from build123d import *

# Parameters (mm, degrees)
BRIDA_BASE1_DEPTH                   = 2.5
CROQUIS16_W                         = 1.5
CROQUIS16_H                         = 11
CORTAR_EXTRUIR1_DEPTH               = 48.758002549
CROQUIS17_W                         = 1.5
CROQUIS17_H                         = 11
CORTAR_EXTRUIR2_DEPTH               = 48.758002549
CROQUIS18_R                         = 2
SALIENTE_EXTRUIR1_DEPTH             = 1.5
CROQUIS19_R                         = 2.7
SALIENTE_EXTRUIR2_DEPTH             = 4.5
CROQUIS20_R                         = 2.7
SALIENTE_EXTRUIR3_DEPTH             = 4.5
CROQUIS21_R                         = 2
SALIENTE_EXTRUIR4_DEPTH             = 1.5
DI_METRO_DE_TALADRO_3_0_3_1_D       = 3
DI_METRO_DE_TALADRO_3_0_3_2_D       = 3
DI_METRO_DE_TALADRO_3_0_3_2_DEPTH   = 8.5
DI_METRO_DE_TALADRO_7_2_7_2_1_D     = 7.2
DI_METRO_DE_TALADRO_7_2_7_2_1_DEPTH = 4
DI_METRO_DE_TALADRO_3_0_3_3_D       = 3
DI_METRO_DE_TALADRO_3_0_3_3_DEPTH   = 8.5
DI_METRO_DE_TALADRO_5_0_5_1_D       = 5
DI_METRO_DE_TALADRO_5_0_5_1_DEPTH   = 7
PLIEGUE_START                       = -35.363495408
PLIEGUE_CROQUIZADO1_OUTLINE_W       = 17
PLIEGUE_CROQUIZADO1_OUTLINE_H       = 2.5
PLIEGUE_CROQUIZADO1_DEPTH           = 19.863495408
PLIEGUE_START_2                     = -15.5
PLIEGUE_CROQUIZADO1_2_DEPTH         = 2.5
PLIEGUE_START_3                     = 15
PLIEGUE_CROQUIZADO1_3_DEPTH         = 18
PLIEGUE_CROQUIZADO2_OUTLINE_W       = 17
PLIEGUE_CROQUIZADO2_OUTLINE_H       = 2.5
PLIEGUE_CROQUIZADO2_DEPTH           = 19.863495408
PLIEGUE_CROQUIZADO2_2_DEPTH         = 2.5
PLIEGUE_START_4                     = -33
PLIEGUE_CROQUIZADO2_3_DEPTH         = 18


with BuildPart() as part:
    # Brida base1: sheet metal written as solids
    # Croquis11 → Brida base1 (new body)
    with BuildSketch(Plane.XY.offset(2.5)):
        with BuildLine():
            Line((-30, -35.363495408), (-17, -35.363495408))
            ThreePointArc((-17, -35.363495408), (-15.585786438, -34.777708971), (-15, -33.363495408))
            Line((-15, -33.363495408), (-15, -12.875))
            Line((-15, -12.875), (-14.875, -12.875))
            Line((-14.875, -12.875), (-14.875, -15.5))
            Line((-14.875, -15.5), (-12, -15.5))
            Line((-12, -15.5), (-12, -20))
            ThreePointArc((-12, -20), (0, -32), (12, -20))
            Line((12, -20), (12, -15.5))
            Line((12, -15.5), (14.875, -15.5))
            Line((14.875, -15.5), (14.875, -12.875))
            Line((14.875, -12.875), (15, -12.875))
            Line((15, -12.875), (15, -33.363495408))
            ThreePointArc((15, -33.363495408), (15.585786438, -34.777708971), (17, -35.363495408))
            Line((17, -35.363495408), (30, -35.363495408))
            ThreePointArc((30, -35.363495408), (31.414213562, -34.777708971), (32, -33.363495408))
            Line((32, -33.363495408), (32, 22))
            ThreePointArc((32, 22), (29.071067812, 29.071067812), (22, 32))
            Line((22, 32), (-22, 32))
            ThreePointArc((-22, 32), (-29.071067812, 29.071067812), (-32, 22))
            Line((-32, 22), (-32, -33.363495408))
            ThreePointArc((-32, -33.363495408), (-31.414213562, -34.777708971), (-30, -35.363495408))
        make_face()
    extrude(amount=-BRIDA_BASE1_DEPTH)

    # Croquis16 → Cortar-Extruir1 (cut, through all)
    with BuildSketch(Plane.XY.offset(2.5)):
        with Locations((-20.75, -29.863495408)):
            Rectangle(CROQUIS16_W, CROQUIS16_H)
    extrude(amount=-CORTAR_EXTRUIR1_DEPTH, mode=Mode.SUBTRACT)

    # Croquis17 → Cortar-Extruir2 (cut, through all)
    with BuildSketch(Plane(origin=(0, 0, 0), x_dir=(-1, 0, 0), z_dir=(0, 0, -1))):
        with Locations((-20.75, -29.863495408)):
            Rectangle(CROQUIS17_W, CROQUIS17_H)
    extrude(amount=-CORTAR_EXTRUIR2_DEPTH, mode=Mode.SUBTRACT)

    # Croquis18 → Saliente-Extruir1 (add)
    with BuildSketch(Plane(origin=(0, 0, 0), x_dir=(-1, 0, 0), z_dir=(0, 0, -1))):
        with Locations(Location((1.5, 17.65, 0), (0, 0, 180))):
            Circle(CROQUIS18_R)
    extrude(amount=SALIENTE_EXTRUIR1_DEPTH)

    # Croquis19 → Saliente-Extruir2 (add)
    with BuildSketch(Plane.XY.offset(2.5)):
        with Locations((23.5, 7.55)):
            Circle(CROQUIS19_R)
    extrude(amount=SALIENTE_EXTRUIR2_DEPTH)

    # Croquis20 → Saliente-Extruir3 (add)
    with BuildSketch(Plane.XY.offset(2.5)):
        with Locations((9.5, 7.55)):
            Circle(CROQUIS20_R)
    extrude(amount=SALIENTE_EXTRUIR3_DEPTH)

    # Croquis21 → Saliente-Extruir4 (add)
    with BuildSketch(Plane(origin=(0, 0, 0), x_dir=(-1, 0, 0), z_dir=(0, 0, -1))):
        with Locations(Location((19, -1.25, 0), (0, 0, 180))):
            Circle(CROQUIS21_R)
    extrude(amount=SALIENTE_EXTRUIR4_DEPTH)

    # Diámetro de taladro Ø3.0 (3)1 (through all)
    with Locations(Plane.XY.offset(2.5)):
        with Locations((-19, -1.25)):
            Hole(DI_METRO_DE_TALADRO_3_0_3_1_D / 2)

    # Diámetro de taladro Ø3.0 (3)2
    with Locations(Plane.XY.offset(7)):
        with Locations((23.5, 7.55), (9.5, 7.55)):
            Hole(DI_METRO_DE_TALADRO_3_0_3_2_D / 2, depth=DI_METRO_DE_TALADRO_3_0_3_2_DEPTH)

    # Diámetro de taladro Ø7.2 (7.2)1
    with Locations(Plane.XY.offset(2.5)):
        with Locations((0, -20.1)):
            Hole(DI_METRO_DE_TALADRO_7_2_7_2_1_D / 2, depth=DI_METRO_DE_TALADRO_7_2_7_2_1_DEPTH)

    # Diámetro de taladro Ø3.0 (3)3
    with Locations(Plane(origin=(0, 0, -1.5), x_dir=(-1, 0, 0), z_dir=(0, 0, -1))):
        with Locations((1.5, 17.65)):
            Hole(DI_METRO_DE_TALADRO_3_0_3_3_D / 2, depth=DI_METRO_DE_TALADRO_3_0_3_3_DEPTH)

    # Diámetro de taladro Ø5.0 (5)1
    with Locations(Plane(origin=(0, 0, 0), x_dir=(-1, 0, 0), z_dir=(0, 0, -1))):
        with Locations((20, 20.1), (-20, 20.1)):
            Hole(DI_METRO_DE_TALADRO_5_0_5_1_D / 2, depth=DI_METRO_DE_TALADRO_5_0_5_1_DEPTH)

    # Pliegue croquizado1: read off the stored shape, not the designer's step
    # Pliegue croquizado1 outline → Pliegue croquizado1 (cut)
    with BuildSketch(Plane(origin=(0, 0, 0), x_dir=(1, 0, 0), z_dir=(0, 1, 0)).offset(PLIEGUE_START)):
        with Locations((23.5, -1.25)):
            Rectangle(PLIEGUE_CROQUIZADO1_OUTLINE_W, PLIEGUE_CROQUIZADO1_OUTLINE_H)
    extrude(amount=PLIEGUE_CROQUIZADO1_DEPTH, mode=Mode.SUBTRACT)

    # Pliegue croquizado1 2 outline → Pliegue croquizado1 2 (add)
    with BuildSketch(Plane(origin=(0, 0, 0), x_dir=(1, 0, 0), z_dir=(0, 1, 0)).offset(PLIEGUE_START_2)):
        with BuildLine():
            Line((15, 0), (32, 0))
            Line((32, 0), (32, 18.4))
            ThreePointArc((32, 18.4), (31.414213562, 19.814213562), (30, 20.4))
            Line((30, 20.4), (21.5, 20.4))
            Line((21.5, 20.4), (21.5, 9.4))
            Line((21.5, 9.4), (20, 9.4))
            Line((20, 9.4), (20, 20.4))
            Line((20, 20.4), (17, 20.4))
            ThreePointArc((17, 20.4), (15.585786438, 19.814213562), (15, 18.4))
            Line((15, 18.4), (15, 0))
        make_face()
    extrude(amount=PLIEGUE_CROQUIZADO1_2_DEPTH)

    # Pliegue croquizado1 3 outline → Pliegue croquizado1 3 (cut)
    with BuildSketch(Plane.YZ.offset(PLIEGUE_START_3)):
        with BuildLine():
            Line((-15.5, 2.5), (-15.5, 0))
            ThreePointArc((-15.5, 0), (-14.767766953, 1.767766953), (-13, 2.5))
            Line((-13, 2.5), (-15.5, 2.5))
        make_face()
    extrude(amount=PLIEGUE_CROQUIZADO1_3_DEPTH, mode=Mode.SUBTRACT)

    # Pliegue croquizado2: read off the stored shape, not the designer's step
    # Pliegue croquizado2 outline → Pliegue croquizado2 (cut)
    with BuildSketch(Plane(origin=(0, 0, 0), x_dir=(1, 0, 0), z_dir=(0, 1, 0)).offset(PLIEGUE_START)):
        with Locations((-23.5, -1.25)):
            Rectangle(PLIEGUE_CROQUIZADO2_OUTLINE_W, PLIEGUE_CROQUIZADO2_OUTLINE_H)
    extrude(amount=PLIEGUE_CROQUIZADO2_DEPTH, mode=Mode.SUBTRACT)

    # Pliegue croquizado2 2 outline → Pliegue croquizado2 2 (add)
    with BuildSketch(Plane(origin=(0, 0, 0), x_dir=(1, 0, 0), z_dir=(0, 1, 0)).offset(PLIEGUE_START_2)):
        with BuildLine():
            ThreePointArc((-30, 20.4), (-31.414213562, 19.814213562), (-32, 18.4))
            Line((-32, 18.4), (-32, 0))
            Line((-32, 0), (-15, 0))
            Line((-15, 0), (-15, 18.4))
            ThreePointArc((-15, 18.4), (-15.585786438, 19.814213562), (-17, 20.4))
            Line((-17, 20.4), (-20, 20.4))
            Line((-20, 20.4), (-20, 9.4))
            Line((-20, 9.4), (-21.5, 9.4))
            Line((-21.5, 9.4), (-21.5, 20.4))
            Line((-21.5, 20.4), (-30, 20.4))
        make_face()
    extrude(amount=PLIEGUE_CROQUIZADO2_2_DEPTH)

    # Pliegue croquizado2 3 outline → Pliegue croquizado2 3 (cut)
    with BuildSketch(Plane.YZ.offset(PLIEGUE_START_4)):
        with BuildLine():
            Line((-15.5, 2.5), (-15.5, 0))
            ThreePointArc((-15.5, 0), (-14.767766953, 1.767766953), (-13, 2.5))
            Line((-13, 2.5), (-15.5, 2.5))
        make_face()
    extrude(amount=PLIEGUE_CROQUIZADO2_3_DEPTH, mode=Mode.SUBTRACT)


solid = part.part
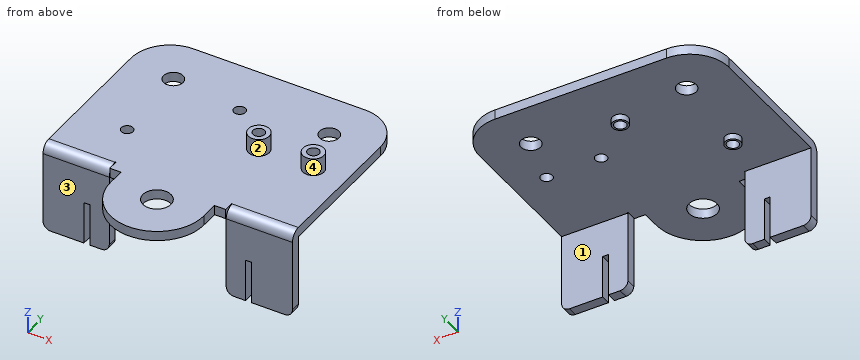
CAD build for the part. Positions are in the model's coordinates, mm. Face numbers are marked on the shaded views. A direction names the side the tool comes from. Coordinates: 2 decimals unless noted, no trailing zeros. Loops run counter-clockwise (first coordinate to the right, second up) from the corner with the lowest first, then second, coordinate; pieces in that order, holes last. Notation, with made-up numbers: (-15, 7.5) - (17, 7.5) arc R24 cw to (17, 40.5) - close; hole circle Ø3 at (64.5, -37). An arc over 180 degrees is marked (long way). Use one line per item in the form item = value. Start each with the question number.
1) Band-saw the part on A-A (z = -11.5). Give the cut face in (x, y).
2) Two-plate mould, pull along X, no slides. Class the marked faces 1 and 2: +X half, -X half, draft (parallel to the pull), parting line (faces both ways), or undercut.
3) Drill centre lines: L1, parallel to Y at x = 9.5, z = 4; L2, parallel to Y at x = -1.5, z = -0.1; L3, parallel to Y at x = -20, z = 1.15. Where is each one in solid material? Low to high. Write a range as from..to.
4) Flat gauge pins, fed straight in: pin 1 (10 mm diameter, centred on x = 23.5, y = 25, fed in from +Z); pin 2 (2 mm diameter, centred on x = 18, z = -15.5, fed in from +Y); pin 3 (0.8 mm diameter, centred on x = -21, y = -14.5, fed in from -Z); pin 4 (6.5 mm diameter, centred on x = 0, y = -20.1, fed in from +Z). Where does each tip first touch, or does it go through?
5) Band-saw the part on D-D (x = -18.5). Give the cut face in (y, z), and give its area (3 significant figures).
6) Band-saw the part on B-B (y = 7.55). Give the cut face in (x, z), and give its area (3 significant figures).
7) Tool access for the marked faces 3 and 4: list every direction of +Z, -Z, +X, -X, +Y, -Y with a clear straight run to the whole face (end or side of a thin tool).
8) Band-saw the part on C-C (x = 23.5). Give the cut face in (y, z), and give its area (3 significant figures).
Check values:
q1.outline = (-32, -15.5) - (-21.5, -15.5) - (-21.5, -13) - (-32, -13) - close; (-20, -15.5) - (-15, -15.5) - (-15, -13) - (-20, -13) - close; (15, -15.5) - (20, -15.5) - (20, -13) - (15, -13) - close; (21.5, -15.5) - (32, -15.5) - (32, -13) - (21.5, -13) - close
q2.face_1 = draft
q2.face_2 = undercut
q3.L1 = 4.85..6.05, 9.05..10.25
q3.L2 = 15.65..16.15, 19.15..19.65
q3.L3 = -15.22..-2.37, -0.13..17.6, 22.6..32
q4.pin_1 = 2.5
q4.pin_2 = -13
q4.pin_3 = -9.4
q4.pin_4 = through
q5.outline = (-15.5, -20.4) - (-13, -20.4) - (-13, 0) - (-3.19, 0) - (-3.19, -1.5) - (-2.66, -1.5) - (-2.66, 2.5) - (-13, 2.5) arc R2.5 ccw to (-15.5, 0) - close; (0.16, -1.5) - (0.69, -1.5) - (0.69, 0) - (18.1, 0) - (18.1, 2.5) - (0.16, 2.5) - close; (22.1, 0) - (32, 0) - (32, 2.5) - (22.1, 2.5) - close
q5.area = 153 mm2
q6.outline = (-32, 0) - (8, 0) - (8, 7) - (6.8, 7) - (6.8, 2.5) - (-32, 2.5) - close; (11, 0) - (22, 0) - (22, 7) - (20.8, 7) - (20.8, 2.5) - (12.2, 2.5) - (12.2, 7) - (11, 7) - close; (25, 0) - (32, 0) - (32, 2.5) - (26.2, 2.5) - (26.2, 7) - (25, 7) - close
q6.area = 167 mm2
q7.face_3 = +Z, -Z, +X, -X, -Y
q7.face_4 = +Z
q8.outline = (-15.5, -20.4) - (-13, -20.4) - (-13, 0) - (6.05, 0) - (6.05, 7) - (4.85, 7) - (4.85, 2.5) - (-13, 2.5) arc R2.5 ccw to (-15.5, 0) - close; (9.05, 0) - (31.89, 0) - (31.89, 2.5) - (10.25, 2.5) - (10.25, 7) - (9.05, 7) - close
q8.area = 171 mm2
